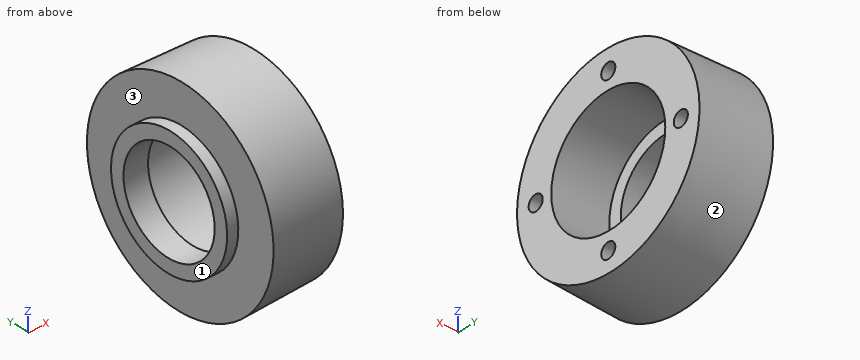
from build123d import *

# Parameters (mm, degrees)
DAIRESEL_KAPLAMA1_COUNT = 4


with BuildPart() as part:
    # Çizim2 → Döndür1 (revolve)
    with BuildSketch(Plane.XY, mode=Mode.PRIVATE) as d_nd_r1_sk:
        Polygon((0, 22), (11, 22), (11, 27.5), (37, 27.5), (37, 44), (5, 45), (5, 28), (0, 28), align=None)
    revolve(d_nd_r1_sk.sketch.rotate(Axis((0, 0, 0), (1, 0, 0)), 90), axis=Axis((0, 0, 0), (1, 0, 0)))

    # Çizim5 → M8 Dişli Delik1 (revolve, cut)
    with BuildSketch(Plane(origin=(37, 35, 0), x_dir=(0, 0, -1), z_dir=(0, 1, 0))):
        Polygon((0, 0), (0, 24.292926105), (3.4, 22.25), (3.4, 0), align=None)
    m8_di_li_delik1 = revolve(axis=Axis((43.35, 35, 0), (-1, 0, 0)), mode=Mode.SUBTRACT)

    # Dairesel Kaplama1: M8 Dişli Delik1 ×4 about axis
    dairesel_kaplama1_axis = Axis((0, 0, 0), (1, 0, 0))
    for i in range(1, DAIRESEL_KAPLAMA1_COUNT):
        add(m8_di_li_delik1.rotate(dairesel_kaplama1_axis, i * 360 / DAIRESEL_KAPLAMA1_COUNT), mode=Mode.SUBTRACT)


solid = part.part
Design review of the part built by this model. Coordinates are the model's own, in mm. Face numbers are marked on the shaded views. A direction names the side the tool comes from. Give positions to 0.01 mm unless a question says otherwise; leave off trailing zeros. Order: outer loops, then holes, each group sorted by start corner. A loop starts at its lowest first (then second) coordinate and runs counter-clockwise, first axis right, second up. Notation, with made-up numbers: (68, 30) - (99, 30) arc R19 ccw to (99, 49) - close; hole circle Ø2 at (59.25, -23). An arc over 180 degrees is marked (long way). Write item = value, one per line. Start each with the question number.
Q1. Tool access review of the marked faces 1, 2 and 3: name each direction out of +Z, -Z, +X, -X, +Y, -Y from which nothing blocks a thin tool from reaching the whole face with its end or side.
Q2. We need section A-A on x = 25. State the section outline as (y, z) points (3 decimals), plus the area to 3 significant figures.
Q3. To check wall thickness, follow L1, parallel to Y at x = 27, z = 0; L2, parallel to Y at x = 18, z = 0; L3, parallel to X at y = -19, z = 18.5. State the ranges of each line that lie inside material, in increasing order. Write a range as from..to.
Q4. We need section B-B on x = 7. State the section outline as (y, z) points (1 decimal).
Q5. Clearance check with flat-ended pins moving along their axes: pin 1 Ø4 at (y, z) = (35, 0) entering from +X; pin 2 Ø1 at (x, z) = (16, 16.5) entering from +Y; pin 3 Ø8 at (y, z) = (-35, 0) entering from +X; pin 4 Ø1.5 at (x, z) = (24.5, 33.5) entering from +Y. State where each tip first meets the part, or that it passes through.
Working result:
q1.face_1 = +Z, -Z, -X, +Y, -Y
q1.face_2 = +X
q1.face_3 = -X
q2.outline = circle Ø88.75 at (0, 0); hole circle Ø6.8 at (-35, 0); hole circle Ø55 at (0, 0); hole circle Ø6.8 at (0, -35); hole circle Ø6.8 at (0, 35); hole circle Ø6.8 at (35, 0)
q2.area = 3,670 mm²
q3.L1 = -44.31..-38.4, -31.6..-27.5, 27.5..31.6, 38.4..44.31
q3.L2 = -44.59..-38.4, -31.6..-27.5, 27.5..31.6, 38.4..44.59
q3.L3 = 0..11
q4.outline = circle Ø89.9 at (0, 0); hole circle Ø44 at (0, 0)
q5.pin_1 = 13.91
q5.pin_2 = 41.69
q5.pin_3 = 37
q5.pin_4 = 29.97
